Work out the finished part from the listing and answer in its coordinate system (mm). A direction names the side the tool comes from. Give positions to 0.01 mm unless a question says otherwise; leave off trailing zeros. Loops run counter-clockwise (first coordinate to the right, second up) from the corner with the lowest first, then second, coordinate; pieces in that order, holes last. Notation, with made-up numbers: (-24, -37) - (-19, -37) arc R16 cw to (-19, -15) - close; hole circle Ø7 at (29, 24). An arc over 180 degrees is marked (long way). One line per question, with ' | ' between items. Start each with the question number.
1. For a pull along Z with two mould halves and no side action, classify faces 4 (the face through (10.541, 5.07, -143.283)), 5 (the face through (10, 0, -80)), 6 (the face through (0.17, 2.8, -4.32)) as released by +Z, released by -Z, zero draft, split by the parting line, or undercut.
2. Each of these flat-tipped pins is pushed along its axis until it touches: pin 1 (6 mm diameter, centred on y = -2.5, z = -105, fed in from -X); pin 2 (3 mm diameter, centred on y = -5.5, z = -16.5, fed in from -X); pin 3 (5.5 mm diameter, centred on x = 7, z = -69, fed in from -Y). Where does it stop, or does it pass through?
3. Section B-B (y = -10) is taken. Determine the outline of the cut face in (x, z), plus the area to 3 significant figures.
4. Find the intervals of material crossed by line 1 (X direction, y = 5, z = -40) (3 decimals); line 2 (X direction, y = 6.25, z = -145); line 3 (Z direction, x = 13.25, y = -10), in increasing order.
5. Section D-D (z = -40) is taken. Determine the outline of the cut face in (x, y) (3 decimals), plus the area to 4 significant figures.
6. Section A-A (z = -145) is taken. Determine the outline of the cut face in (x, y).
7. Section C-C (x = 10) is taken. Give the number of separate pieces and of enclosed holes in the cut face, plus the area to 3 significant figures.
8. Which of the six approach directions +Z, -Z, +X, -X, +Y, -Y give full straight-line access (tool end or side, diameter ignored) to faces 1 (the face through (10, -6, -20)), 2 (the face through (10, -6, -10)), 3 (the face through (5, -6, -15))?
from build123d import *

# Parameters (mm, degrees)
SKETCH1_W                   = 20
SKETCH1_H                   = 150
BOSS_EXTRUDE1_DEPTH         = 10
M3_CLEARANCE_HOLE1_D        = 3.6
SKETCH3_W                   = 10
SKETCH3_H                   = 10
BOSS_EXTRUDE2_DEPTH         = 14
M3_CLEARANCE_HOLE5_D        = 3.6
F_1_4_0_25_DIAMETER_HOLE1_D = 6.35
FILLET1_R                   = 10
FILLET2_R                   = 2
CHAMFER1_SIZE               = 1
FILLET3_R                   = 1
CHAMFER2_SIZE               = 1


with BuildPart() as part:
    # Sketch1 → Boss-Extrude1 (new body)
    with BuildSketch(Plane(origin=(0, 0, 0), x_dir=(1, 0, 0), z_dir=(0, 1, 0))):
        with Locations((10, 75)):
            Rectangle(SKETCH1_W, SKETCH1_H)
    extrude(amount=BOSS_EXTRUDE1_DEPTH)

    # M3 Clearance Hole1 (through all)
    with Locations(Plane(origin=(10, 0, -145), x_dir=(0, 0, -1), z_dir=(0, -1, 0))):
        with Locations((0, 0)):
            Hole(M3_CLEARANCE_HOLE1_D / 2)

    # Sketch3 → Boss-Extrude2 (add)
    with BuildSketch(Plane.XZ):
        with Locations((10, -15)):
            Rectangle(SKETCH3_W, SKETCH3_H)
    extrude(amount=BOSS_EXTRUDE2_DEPTH)

    # M3 Clearance Hole5 (through all)
    with Locations(Plane(origin=(5, -10, -15), x_dir=(0, 0, -1), z_dir=(-1, 0, 0))):
        with Locations((0, 0)):
            Hole(M3_CLEARANCE_HOLE5_D / 2)

    # 1/4 (0.25) Diameter Hole1 (through all)
    with Locations(Plane(origin=(10, 0, -40), x_dir=(0, 0, -1), z_dir=(0, -1, 0))):
        with Locations((0, 0)):
            Hole(F_1_4_0_25_DIAMETER_HOLE1_D / 2)

    # Fillet1
    fillet1_edges = [part.edges().sort_by_distance(p)[0] for p in [
        (10, 0, 0),
    ]]
    fillet(fillet1_edges, radius=FILLET1_R - 0.0001)  # a hair under: the kernel refuses the full size

    # Fillet2
    fillet2_edges = [part.edges().sort_by_distance(p)[0] for p in [
        (10, 10, 0),
    ]]
    fillet(fillet2_edges, radius=FILLET2_R)

    # Chamfer1
    chamfer1_edges = [part.edges().sort_by_distance(p)[0] for p in [
        (20, 0, -79.99995),
        (0, 2.094314553, -3.876198607),
        (20, 10, -76.127005384),
        (0, 10, -76.127005384),
        (20, 2.094314553, -3.876198607),
        (20, 9.224752526, -0.672877867),
        (0, 9.224752526, -0.672877867),
        (0, 0, -79.99995),
        (0, 5, -150),
        (20, 5, -150),
    ]]
    chamfer(chamfer1_edges, length=CHAMFER1_SIZE)

    # Fillet3
    fillet3_edges = [part.edges().sort_by_distance(p)[0] for p in [
        (5, -14, -15),
        (10, -14, -20),
        (15, -14, -15),
        (10, -14, -10),
    ]]
    fillet(fillet3_edges, radius=FILLET3_R)

    # Chamfer2
    chamfer2_edges = [part.edges().sort_by_distance(p)[0] for p in [
        (10, 0, -150),
        (10, 10, -150),
    ]]
    chamfer(chamfer2_edges, length=CHAMFER2_SIZE)


solid = part.part
Conclusion:
1) face 4: undercut | face 5: zero draft | face 6: released by +Z
2) pin 1: x = 0.5 | pin 2: x = 5 | pin 3: y = 0
3) outline: (5, -20) - (15, -20) - (15, -16.8) - (5, -16.8) - close; (5, -13.2) - (15, -13.2) - (15, -10) - (5, -10) - close | area: 64.0 mm²
4) line 1: 0 to 6.825, 13.175 to 20 | line 2: 0 to 8.2, 11.8 to 20 | line 3: -20 to -16.8, -13.2 to -10
5) outline: (0, 1) - (1, 0) - (6.825, 0) - (6.825, 10) - (1, 10) - (0, 9) - close; (13.175, 0) - (19, 0) - (20, 1) - (20, 9) - (19, 10) - (13.175, 10) - close | area: 134.5 mm²
6) outline: (0, 1) - (1, 0) - (8.2, 0) - (8.2, 10) - (1, 10) - (0, 9) - close; (11.8, 0) - (19, 0) - (20, 1) - (20, 9) - (19, 10) - (11.8, 10) - close
7) separate pieces: 3 | enclosed holes: 1 | area: 1,510 mm²
8) face 1: -Z, +X, -X, -Y | face 2: +Z, +X, -X, -Y | face 3: +Z, -Z, -X, -Y
